Geometry: see drawing. Coordinates: mm, zero at the bounding-box minimum. A direction names the side the tool comes from. Coordinates: 2 decimals unless noted, no trailing zeros. Order: outer loops, then holes, each group sorted by start corner. A loop starts at its lowest first (then second) coordinate and runs counter-clockwise, first axis right, second up.
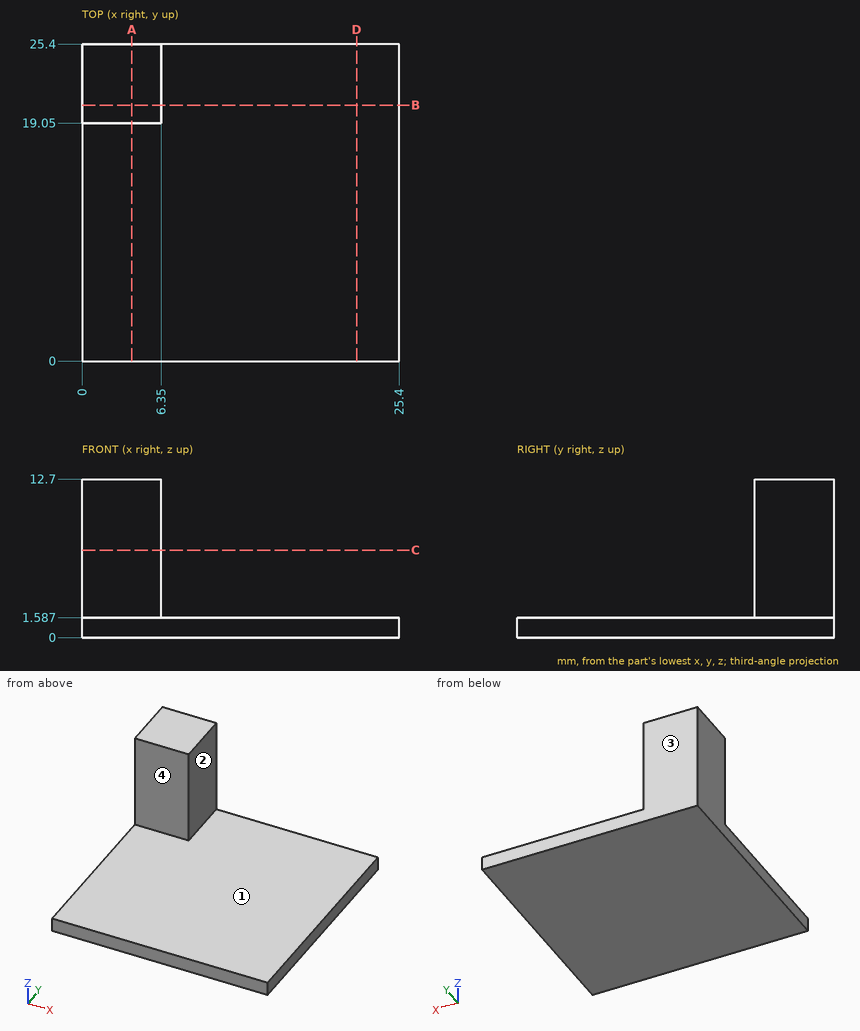
Item 1: Cut plane C-C on z = 7. Return loops of the section in (x, y), then the cut area to 3 significant figures.
Response values:
outline: (0, 19.05) - (6.35, 19.05) - (6.35, 25.4) - (0, 25.4) - close
area: 40.3 mm2
Item 2: Access query for the marked faces 1, 2, 3 and 4. Directions: +Z, -Z, +X, -X, +Y, -Y. A direction counts if a zero-diameter tool reaches every point of the face in a straight line with its end or side. Return the directions, or none.
Response values:
face 1: +Z, +X, -Y
face 2: +Z, +X, +Y, -Y
face 3: +Z, -Z, +X, -X, +Y
face 4: +Z, +X, -X, -Y
Item 3: Cut plane A-A on x = 4. Return loops of the section in (y, z).
Response values:
outline: (0, 0) - (25.4, 0) - (25.4, 12.7) - (19.05, 12.7) - (19.05, 1.59) - (0, 1.59) - close
Item 4: Ray query, probe 1 along Z at (x, y) = (11.75, 17.75); probe 2 along Y at (x, z) = (6.25, 4.75). Return the intervals inside material, ascending.
Response values:
probe 1: z = 0 to 1.59
probe 2: y = 19.05 to 25.4
Item 5: Cut plane D-D on x = 22. Return loops of the section in (y, z).
Response values:
outline: (0, 0) - (25.4, 0) - (25.4, 1.59) - (0, 1.59) - close
Item 6: Cut plane B-B on y = 20.5. Return loops of the section in (x, z), then the cut area to 3 significant figures.
Response values:
outline: (0, 0) - (25.4, 0) - (25.4, 1.59) - (6.35, 1.59) - (6.35, 12.7) - (0, 12.7) - close
area: 111 mm2
Item 7: Pin query (flat end, axial travel): pin 1 Ø3 at (y, z) = (22.5, 9.5) entering from +X; pin 2 Ø1.9 at (x, z) = (4.5, 7.5) entering from -Y; pin 3 Ø3 at (x, z) = (5, 11) entering from -Y; pin 4 Ø1 at (x, y) = (14, 11) entering from -Z. Return the tip coordinate at first contact, or that it passes through.
Response values:
pin 1: stops at x = 6.35
pin 2: stops at y = 19.05
pin 3: stops at y = 19.05
pin 4: stops at z = 0
